Work out the finished part from the listing and answer in its coordinate system (mm). Face numbers are marked on the shaded views. Coordinates: 2 decimals unless noted, no trailing zeros. Write each loop counter-clockwise with the first axis right and the second up, starting at its lowest first coordinate (ties: lowest second). Pieces come first, ordered by that corner, then holes. Notation, with made-up numbers: M -24.75,61 L 3.25,61 A8 cw 3.25,76 Z; hole C -12,-20 d10. An arc over 180 degrees is marked long. Use CSV: the item, a comma, the result in double quotes.
from build123d import *

# Parameters (mm, degrees)
SKETCH1_R           = 21.53
SKETCH1_R_2         = 19.53
BOSS_EXTRUDE1_DEPTH = 197.41
SKETCH2_R           = 11.53
CUT_EXTRUDE1_DEPTH  = 200.744311308


with BuildPart() as part:
    # Sketch1 → Boss-Extrude1 (new body)
    with BuildSketch(Plane(origin=(0, 0, 0), x_dir=(1, 0, 0), z_dir=(0, 1, 0))):
        with Locations(Location((0, 0, 0), (0, 0, 270))):
            Circle(SKETCH1_R)
        with Locations(Location((0, 0, 0), (0, 0, 270))):
            Circle(SKETCH1_R_2, mode=Mode.SUBTRACT)
    extrude(amount=BOSS_EXTRUDE1_DEPTH)

    # Sketch2 → Cut-Extrude1 (cut, through all)
    with BuildSketch(Plane(origin=(0, 0, 0), x_dir=(0, 0, -1), z_dir=(1, 0, 0))):
        with Locations(Location((0, 132.71, 0), (0, 0, 180))):
            Circle(SKETCH2_R)
        with Locations(Location((0, 81.41, 0), (0, 0, 180))):
            Circle(SKETCH2_R)
        with Locations(Location((0, 30.11, 0), (0, 0, 180))):
            Circle(SKETCH2_R)
    extrude(amount=CUT_EXTRUDE1_DEPTH, mode=Mode.SUBTRACT)


solid = part.part
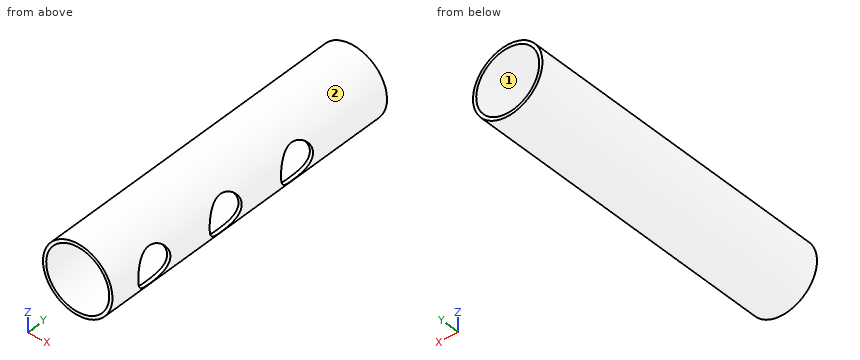
Item 1: For a pull along X with two mould halves and no side action, classify the marked faces 1 and 2 as released by +X, released by -X, zero draft, split by the parting line, or undercut.
Answer:
face 1,"undercut"
face 2,"split by the parting line"
Item 2: The part is cut by section D-D (y = 154). Write down the section's boundary in (x, z), then the cut area to 3 significant figures.
Answer:
outline,"C 0,0 d43.06; hole C 0,0 d39.06"
area,"258 mm2"
Item 3: Consider probe 1 along Y at (x, z) = (19.6, 0); probe 2 along X at (y, z) = (42, -1). Determine where each line is inside the solid, lowest interval first.
Answer:
probe 1,"y = 0 to 18.58, 41.64 to 69.88, 92.94 to 121.18, 144.24 to 197.41"
probe 2,"x = -21.51 to -19.5, 19.5 to 21.51"
Item 4: The part is cut by section B-B (z = 0). Write down the section's boundary in (x, y), then the cut area to 3 significant figures.
Answer:
outline,"M -21.53,0 L -19.53,0 L -19.53,197.41 L -21.53,197.41 Z; M 19.53,0 L 21.53,0 L 21.53,18.58 L 19.53,18.58 Z; M 19.53,41.64 L 21.53,41.64 L 21.53,69.88 L 19.53,69.88 Z; M 19.53,92.94 L 21.53,92.94 L 21.53,121.18 L 19.53,121.18 Z; M 19.53,144.24 L 21.53,144.24 L 21.53,197.41 L 19.53,197.41 Z"
area,"651 mm2"
Item 5: The part is cut by section A-A (x = 0). Write down the section's boundary in (y, z).
Answer:
outline,"M 0,-21.53 L 197.41,-21.53 L 197.41,-19.53 L 0,-19.53 Z; M 0,19.53 L 197.41,19.53 L 197.41,21.53 L 0,21.53 Z"
Item 6: The part is cut by section C-C (z = -14.5). Write down the section's boundary in (x, y).
Answer:
outline,"M -15.92,0 L -13.08,0 L -13.08,197.41 L -15.92,197.41 Z; M 13.08,0 L 15.92,0 L 15.92,197.41 L 13.08,197.41 Z"
Item 7: Given pin 1 (1.5 mm diameter, centred on x = 2.5, y = 72.5, fed in from +Z); pin 2 (10 mm diameter, centred on x = -10.5, y = 55, fed in from +Z); pin 3 (14 mm diameter, centred on y = 132.71, z = 0, fed in from +X), each flat-ended and moving along its own axis, determine where each tip first touches the part or whether it passes through.
Answer:
pin 1,"stops at z = 21.46"
pin 2,"stops at z = 20.82"
pin 3,"stops at x = -18.23"
